Answer from the drawing. Dimensions are ordinates in mm from the lowest x, y and z of the part. Give positions to 0.01 mm unless a question says otherwise; leave off trailing zeros. Write each loop counter-clockwise with the first axis right and the second up, starting at its lowest first coordinate (ties: lowest second). Pieces come first, ordered by that corner, then holes.
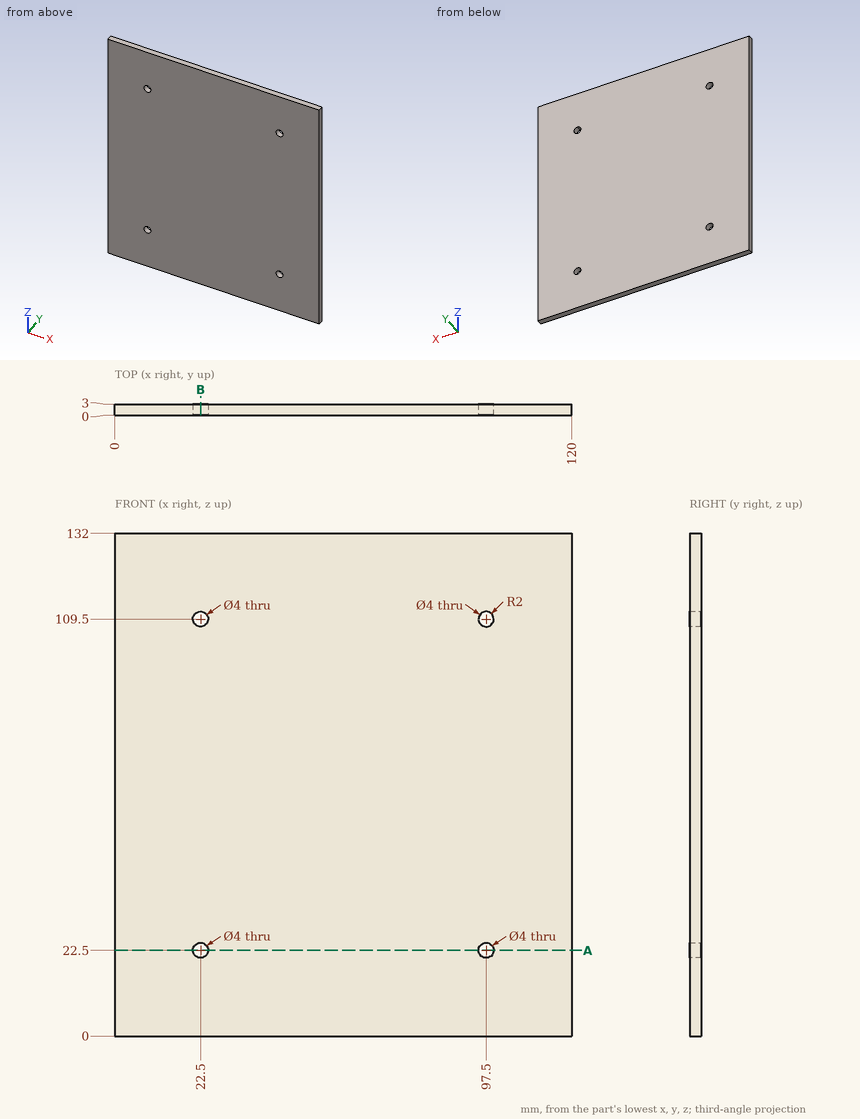
Item 1: Each of these flat-tipped pins is pushed along its axis until it touches: pin 1 Ø6.5 at (x, z) = (97.5, 22.5) entering from -Y; pin 2 Ø2.5 at (x, z) = (22.5, 22.5) entering from -Y. Where does it stop, or does it pass through?
Result set:
pin 1: stops at y = 0
pin 2: passes through
Item 2: Section B-B (x = 22.5) is taken. Write down the section's boundary in (y, z).
Result set:
outline: (0, 0) - (3, 0) - (3, 20.5) - (0, 20.5) - close; (0, 24.5) - (3, 24.5) - (3, 107.5) - (0, 107.5) - close; (0, 111.5) - (3, 111.5) - (3, 132) - (0, 132) - close
Item 3: Section A-A (z = 22.5) is taken. Write down the section's boundary in (x, y), and give its area (3 significant figures).
Result set:
outline: (0, 0) - (20.5, 0) - (20.5, 3) - (0, 3) - close; (24.5, 0) - (95.5, 0) - (95.5, 3) - (24.5, 3) - close; (99.5, 0) - (120, 0) - (120, 3) - (99.5, 3) - close
area: 336 mm2
Item 4: Find the intervals of material crossed by line 1 along X through (y, z) = (2, 22.5); line 2 along Z through (x, y) = (97.5, 2.25), in increasing order.
Result set:
line 1: x = 0 to 20.5, 24.5 to 95.5, 99.5 to 120
line 2: z = 0 to 20.5, 24.5 to 107.5, 111.5 to 132
